Study the drawing (mm; zero at the part's minimum x, y, z) and answer. A direction names the side the tool comes from. Coordinates: 2 decimals unless noted, no trailing zeros. Write each loop counter-clockwise with the first axis right and the second up, starting at its lowest first coordinate (ties: lowest second). Pieces come first, ordered by that corner, then holes. Notation, with made-up numbers: (64, -22.75) - (107, -22.75) arc R24 ccw to (107, 15.25) - close; hole circle Ø11 at (-4, 74.25). An arc over 180 degrees is marked (long way). One line per item, written item: value.
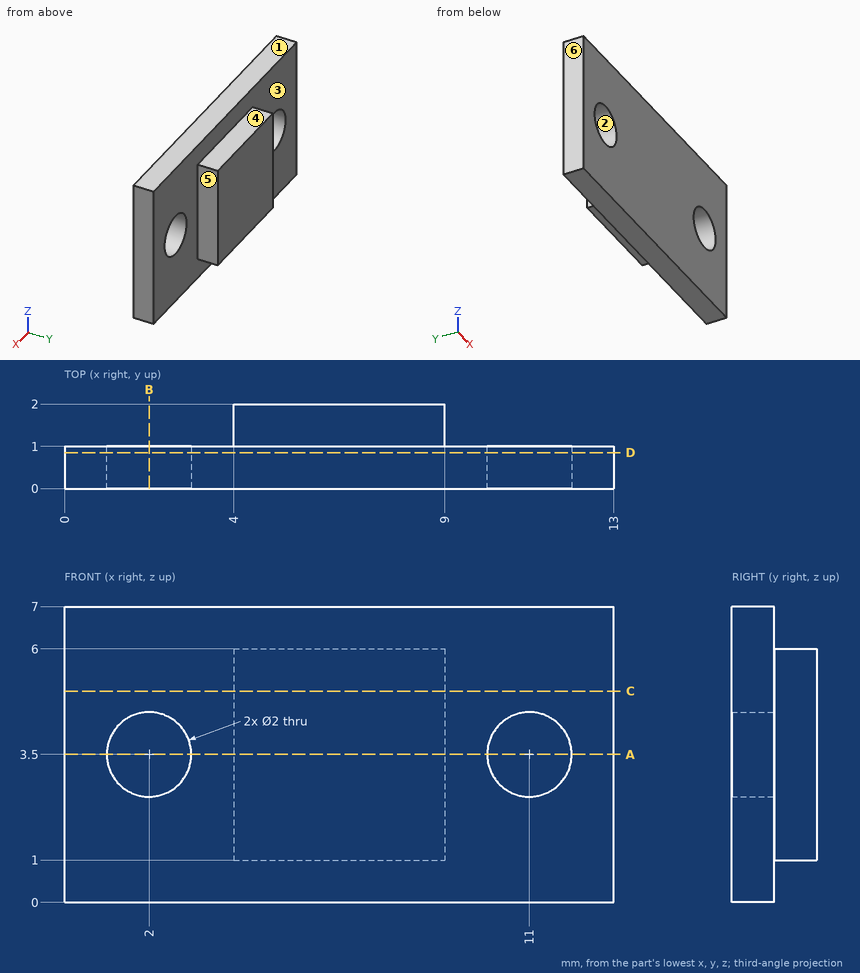
Item 1: Section B-B, the plane x = 2 is taken. Determine the outline of the cut face in (y, z), then the cut area to 3 significant figures.
Evaluation:
outline: (0, 0) - (1, 0) - (1, 2.5) - (0, 2.5) - close; (0, 4.5) - (1, 4.5) - (1, 7) - (0, 7) - close
area: 5.00 mm2
Item 2: Given pin 1 (1 mm diameter, centred on x = 11, z = 1.5, fed in from +Y); pin 2 (0.5 mm diameter, centred on x = 7, y = 1.5, fed in from -Z); pin 3 (0.8 mm diameter, centred on y = 1.5, z = 4, fed in from -X), each flat-ended and moving along its own axis, determine where each tip first touches the part or whether it passes through.
Evaluation:
pin 1: stops at y = 1
pin 2: stops at z = 1
pin 3: stops at x = 4
Item 3: Section A-A, the plane z = 3.5 is taken. Determine the outline of the cut face in (x, y).
Evaluation:
outline: (0, 0) - (1, 0) - (1, 1) - (0, 1) - close; (3, 0) - (10, 0) - (10, 1) - (9, 1) - (9, 2) - (4, 2) - (4, 1) - (3, 1) - close; (12, 0) - (13, 0) - (13, 1) - (12, 1) - close
Item 4: Determine the mould class of the marked faces 1, 2 and 3 for opening direction Z: +Z half, -Z half, draft (parallel to the pull), parting line (faces both ways), or undercut.
Evaluation:
face 1: +Z half
face 2: undercut
face 3: draft
Item 5: Which of the six approach directions +Z, -Z, +X, -X, +Y, -Y give full straight-line access (tool end or side, diameter ignored) to the marked faces 4, 5 and 6?
Evaluation:
face 4: +Z, +X, -X, +Y
face 5: +Z, -Z, +X, +Y
face 6: +Z, -Z, -X, +Y, -Y
Item 6: Consider probe 1 along Z at (x, y) = (11, 0.35); probe 2 along X at (y, z) = (0.4, 3.25); probe 3 along X at (y, z) = (0.6, 2.75). Determine where each line is inside the solid, lowest interval first.
Evaluation:
probe 1: z = 0 to 2.5, 4.5 to 7
probe 2: x = 0 to 1.03, 2.97 to 10.03, 11.97 to 13
probe 3: x = 0 to 1.34, 2.66 to 10.34, 11.66 to 13
Item 7: Section C-C, the plane z = 5 is taken. Determine the outline of the cut face in (x, y), then the cut area to 3 significant figures.
Evaluation:
outline: (0, 0) - (13, 0) - (13, 1) - (9, 1) - (9, 2) - (4, 2) - (4, 1) - (0, 1) - close
area: 18.0 mm2
Item 8: Section D-D, the plane y = 0.85 is taken. Determine the outline of the cut face in (x, z), then the cut area to 3 significant figures.
Evaluation:
outline: (0, 0) - (13, 0) - (13, 7) - (0, 7) - close; hole circle Ø2 at (2, 3.5); hole circle Ø2 at (11, 3.5)
area: 84.7 mm2
